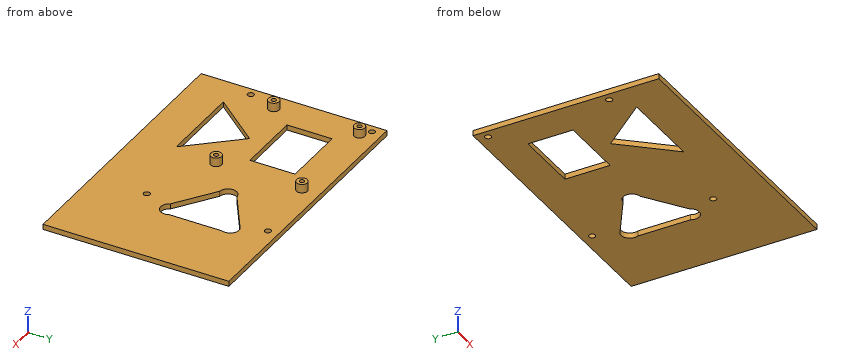
```python
from build123d import *

# Parameters (mm, degrees)
SKETCH001_W   = 159.247498
SKETCH001_H   = 106.166245
SKETCH001_R   = 1.8
SKETCH001_W_2 = 37.327541
SKETCH001_H_2 = 25.790894
PAD_DEPTH     = 3
SKETCH_R      = 3.1
SKETCH_R_2    = 1.35
PAD004_DEPTH  = 5


with BuildPart() as part:
    # Sketch001 → Pad (new body)
    with BuildSketch(Plane.XY):
        with Locations((69.623749, -43.083122)):
            Rectangle(SKETCH001_W, SKETCH001_H)
        with Locations((-5.373725, 3.997676)):
            Circle(SKETCH001_R, mode=Mode.SUBTRACT)
        with Locations((99.381157, 3.997676)):
            Circle(SKETCH001_R, mode=Mode.SUBTRACT)
        with Locations((-5.373725, -65.174667)):
            Circle(SKETCH001_R, mode=Mode.SUBTRACT)
        with Locations((99.381157, -65.174667)):
            Circle(SKETCH001_R, mode=Mode.SUBTRACT)
        with Locations((28.66377, -22.895447)):
            Rectangle(SKETCH001_W_2, SKETCH001_H_2, mode=Mode.SUBTRACT)
        with BuildLine():
            Line((102.543606, -10.170694), (79.745988, -24.831094))
            ThreePointArc((79.745988, -24.831094), (74.954831, -29.68213), (79.457328, -34.802214))
            Line((79.457328, -34.802214), (101.639507, -50.378146))
            ThreePointArc((101.639507, -50.378146), (108.410837, -52.766648), (110.587478, -45.924273))
            Line((110.587478, -45.924273), (110.587478, -15.797321))
            ThreePointArc((110.587478, -15.797321), (108.884887, -9.668253), (102.543606, -10.170694))
        make_face(mode=Mode.SUBTRACT)
        Polygon((30.043512, -45.812858), (7.166186, -73.730591), (54.611111, -73.730591), align=None, mode=Mode.SUBTRACT)
    extrude(amount=PAD_DEPTH)

    # Sketch (on Face23 of Pad) → Pad004 (join)
    with BuildSketch(Plane.XY.offset(3)):
        Circle(SKETCH_R)
        Circle(SKETCH_R_2, mode=Mode.SUBTRACT)
        with Locations((58, 0)):
            Circle(SKETCH_R)
        with Locations((58, 0)):
            Circle(SKETCH_R_2, mode=Mode.SUBTRACT)
        with Locations((0, -49)):
            Circle(SKETCH_R)
        with Locations((0, -49)):
            Circle(SKETCH_R_2, mode=Mode.SUBTRACT)
        with Locations((58, -49)):
            Circle(SKETCH_R)
        with Locations((58, -49)):
            Circle(SKETCH_R_2, mode=Mode.SUBTRACT)
    extrude(amount=PAD004_DEPTH)


solid = part.part
```
Geometry check sheet. Reference: the model listing, model coordinates, mm. Round coordinates to 2 decimals unless told otherwise and drop trailing zeros. Order: outer loops, then holes, each group sorted by start corner. A loop starts at its lowest first (then second) coordinate and runs counter-clockwise, first axis right, second up. Notation, with made-up numbers: (84, -4.5) - (117, -4.5) arc R20 cw to (117, 15.5) - close; hole circle Ø11 at (12.5, -2.75). An arc over 180 degrees is marked (long way). Use a Markdown table: item, result. Add a question column.
1) Section check C-C (y = -72). Record the cut outline in (x, z).
2) Section check B-B (x = 37.5). Record the cut outline in (y, z).
3) Thickness scan on line 1 along Y through (x, z) = (58, 5.35); line 2 along Y through (x, z) = (47, 1.75); line 3 along X through (y, z) = (-48.5, 7.75). Record the ranges inside material, lowest first.
4) Section check D-D (x = 137). Record the cut outline in (y, z).
5) Section check A-A (z = 1.5). Record the cut outline in (x, y), then the cut area to 3 significant figures.
6) Gauge pin test, flat end, axial feed: P1, Ø2, axis at x = -5.37, y = -65.17, coming from the -Z side (3 decimals). Record the tip position at first contact, or that the pin passes through.
Established:
| question | item | result |
|---|---|---|
| 1 | outline | (-10, 0) - (8.58, 0) - (8.58, 3) - (-10, 3) - close; (53.09, 0) - (149.25, 0) - (149.25, 3) - (53.09, 3) - close |
| 2 | outline | (-96.17, 0) - (-73.73, 0) - (-73.73, 3) - (-96.17, 3) - close; (-54.29, 0) - (-35.79, 0) - (-35.79, 3) - (-54.29, 3) - close; (-10, 0) - (10, 0) - (10, 3) - (-10, 3) - close |
| 3 | line 1 | -52.1 to -50.35, -47.65 to -45.9, -3.1 to -1.35, 1.35 to 3.1 |
| 3 | line 2 | -96.17 to -73.73, -65.08 to -35.79, -10 to 10 |
| 3 | line 3 | -3.06 to -1.25, 1.25 to 3.06, 54.94 to 56.75, 59.25 to 61.06 |
| 4 | outline | (-96.17, 0) - (10, 0) - (10, 3) - (-96.17, 3) - close |
| 5 | outline | (-10, -96.17) - (149.25, -96.17) - (149.25, 10) - (-10, 10) - close; hole circle Ø3.6 at (-5.37, -65.17); hole circle Ø3.6 at (-5.37, 4); hole (7.17, -73.73) - (54.61, -73.73) - (30.04, -45.81) - close; hole (10, -35.79) - (47.33, -35.79) - (47.33, -10) - (10, -10) - close; hole (79.46, -34.8) - (101.64, -50.38) arc R5 ccw (long way) to (110.59, -45.92) - (110.59, -15.8) arc R5 ccw to (102.54, -10.17) - (79.75, -24.83) arc R5 ccw to start; hole circle Ø3.6 at (99.38, -65.17); hole circle Ø3.6 at (99.38, 4) |
| 5 | area | 14,300 mm2 |
| 6 | P1 | through |
